Could you check a few things on this model? Use its own coordinates, in mm. A direction names the side the tool comes from. Round coordinates to 2 decimals unless told otherwise and drop trailing zeros. Order: outer loops, then holes, each group sorted by start corner. A loop starts at its lowest first (then second) coordinate and runs counter-clockwise, first axis right, second up.
```python
from build123d import *

# Parameters (mm, degrees)
BOSS_EXTRUDE1_DEPTH = 40
SKETCH2_R           = 10
BOSS_EXTRUDE2_DEPTH = 2
SKETCH3_R           = 1
BOSS_EXTRUDE3_DEPTH = 25.4


with BuildPart() as part:
    # Sketch1 → Boss-Extrude1 (new body)
    with BuildSketch(Plane(origin=(0, 0, 0), x_dir=(1, 0, 0), z_dir=(0, 1, 0))):
        with BuildLine():
            Line((11.5, 21.5), (-11.5, 21.5))
            ThreePointArc((-11.5, 21.5), (-18.571067812, 18.571067812), (-21.5, 11.5))
            Line((-21.5, 11.5), (-21.5, -11.5))
            ThreePointArc((-21.5, -11.5), (-18.571067812, -18.571067812), (-11.5, -21.5))
            Line((-11.5, -21.5), (11.5, -21.5))
            ThreePointArc((11.5, -21.5), (18.571067812, -18.571067812), (21.5, -11.5))
            Line((21.5, -11.5), (21.5, 11.5))
            ThreePointArc((21.5, 11.5), (18.571067812, 18.571067812), (11.5, 21.5))
        make_face()
    extrude(amount=BOSS_EXTRUDE1_DEPTH)

    # Sketch2 → Boss-Extrude2 (add)
    with BuildSketch(Plane(origin=(0, 40, 0), x_dir=(1, 0, 0), z_dir=(0, 1, 0))):
        with Locations(Location((0, 0, 0), (0, 0, 270))):
            Circle(SKETCH2_R)
    extrude(amount=BOSS_EXTRUDE2_DEPTH)

    # Sketch3 → Boss-Extrude3 (add)
    with BuildSketch(Plane(origin=(0, 42, 0), x_dir=(1, 0, 0), z_dir=(0, 1, 0))):
        with Locations(Location((0, 0, 0), (0, 0, 270))):
            Circle(SKETCH3_R)
    extrude(amount=BOSS_EXTRUDE3_DEPTH)


solid = part.part
```
Q1. I need wall thicknesses on L1, parallel to Y at x = 11.5, z = 13.5; L2, parallel to Y at x = 3.5, z = 8; L3, parallel to X at y = 27, z = 12. Which ranges of each line are inside material? Lowest first, please.
Q2. For faces 1 (the flat face through (21.5, 20, 0)), 2 (the cylindrical face through (-1, 55, 0)), which set-ups out of +Z, -Z, +X, -X, +Y, -Y let a thin tool reach every point of the face, with its end or its side?
Q3. For P1, Ø4, axis at x = 16, z = 12, coming from the +Y side; P2, Ø8, axis at x = -2, z = 12, coming from the +Y side, each with a flat end and sliding along its axis, tell me the tip position at first contact or that it passes through.
Q4. Imagine slicing it at C-C, the plane y = 4. Please give me the cut outline in (x, z), then the cut area to 3 significant figures.
Q5. Imagine slicing it at D-D, the plane x = 9. Please give me the cut outline in (y, z), then the cut area to 3 significant figures.
Q6. Imagine slicing it at B-B, the plane x = 0. Please give me the cut outline in (y, z), then the cut area to 3 significant figures.
Q7. Imagine slicing it at A-A, the plane z = 0. Please give me the cut outline in (x, y).
Filled in:
1. L1: y = 0 to 40
1. L2: y = 0 to 42
1. L3: x = -21.49 to 21.49
2. face 1: +Z, -Z, +X, +Y, -Y
2. face 2: +Y
3. P1: stops at y = 40
3. P2: stops at y = 42
4. outline: (-21.5, -11.5) arc R10 ccw to (-11.5, -21.5) - (11.5, -21.5) arc R10 ccw to (21.5, -11.5) - (21.5, 11.5) arc R10 ccw to (11.5, 21.5) - (-11.5, 21.5) arc R10 ccw to (-21.5, 11.5) - close
4. area: 1,760 mm2
5. outline: (0, -21.5) - (40, -21.5) - (40, -4.36) - (42, -4.36) - (42, 4.36) - (40, 4.36) - (40, 21.5) - (0, 21.5) - close
5. area: 1,740 mm2
6. outline: (0, -21.5) - (40, -21.5) - (40, -10) - (42, -10) - (42, -1) - (67.4, -1) - (67.4, 1) - (42, 1) - (42, 10) - (40, 10) - (40, 21.5) - (0, 21.5) - close
6. area: 1,810 mm2
7. outline: (-21.5, 0) - (21.5, 0) - (21.5, 40) - (10, 40) - (10, 42) - (1, 42) - (1, 67.4) - (-1, 67.4) - (-1, 42) - (-10, 42) - (-10, 40) - (-21.5, 40) - close
